from build123d import *

# Parameters (mm, degrees)
CROQUIS1_W     = 30
CROQUIS1_H     = 40
CROQUIS1_H_2   = 30
CROQUIS1_W_2   = 40
EXTRUIR1_DEPTH = 30
CROQUIS5_W     = 30
CROQUIS5_H     = 30
EXTRUIR4_DEPTH = 40
CROQUIS2_W     = 30
CROQUIS2_H     = 30
CROQUIS2_W_2   = 24
CROQUIS2_H_2   = 24
EXTRUIR2_DEPTH = 40
CROQUIS3_W     = 30
CROQUIS3_H     = 30
CROQUIS3_W_2   = 24
CROQUIS3_H_2   = 24
EXTRUIR3_DEPTH = 40
CROQUIS7_W     = 30
CROQUIS7_H     = 30
CROQUIS7_W_2   = 24
CROQUIS7_H_2   = 24
EXTRUIR5_DEPTH = 40
VACIADO1_T     = -2


with BuildPart() as part:
    # Croquis1 → Extruir1 (new body)
    with BuildSketch(Plane(origin=(0, 0, 0), x_dir=(1, 0, 0), z_dir=(0, 1, 0))):
        with Locations((0, 35)):
            Rectangle(CROQUIS1_W, CROQUIS1_H)
        Rectangle(CROQUIS1_W, CROQUIS1_H_2)
        with Locations((35, 0)):
            Rectangle(CROQUIS1_W_2, CROQUIS1_H_2)
    extrude(amount=EXTRUIR1_DEPTH)

    # Croquis5 → Extruir4 (add)
    with BuildSketch(Plane.XZ):
        Rectangle(CROQUIS5_W, CROQUIS5_H)
    extrude(amount=EXTRUIR4_DEPTH)

    # Croquis2 → Extruir2 (cut)
    with BuildSketch(Plane(origin=(55, 0, 0), x_dir=(0, 0, -1), z_dir=(1, 0, 0))):
        with Locations((0, 15)):
            Rectangle(CROQUIS2_W, CROQUIS2_H)
        with Locations((0, 15)):
            Rectangle(CROQUIS2_W_2, CROQUIS2_H_2, mode=Mode.SUBTRACT)
    extrude(amount=-EXTRUIR2_DEPTH, mode=Mode.SUBTRACT)

    # Croquis3 → Extruir3 (cut)
    with BuildSketch(Plane(origin=(0, 0, -55), x_dir=(-1, 0, 0), z_dir=(0, 0, -1))):
        with Locations((0, 15)):
            Rectangle(CROQUIS3_W, CROQUIS3_H)
        with Locations((0, 15)):
            Rectangle(CROQUIS3_W_2, CROQUIS3_H_2, mode=Mode.SUBTRACT)
    extrude(amount=-EXTRUIR3_DEPTH, mode=Mode.SUBTRACT)

    # Croquis7 → Extruir5 (cut)
    with BuildSketch(Plane.XZ.offset(40)):
        Rectangle(CROQUIS7_W, CROQUIS7_H)
        Rectangle(CROQUIS7_W_2, CROQUIS7_H_2, mode=Mode.SUBTRACT)
    extrude(amount=-EXTRUIR5_DEPTH, mode=Mode.SUBTRACT)

    # Vaciado1
    vaciado1_openings = [part.faces().sort_by_distance(p)[0] for p in [
        (55, 15, 0),
        (0, 15, -55),
        (0, -40, 0),
    ]]
    offset(amount=VACIADO1_T, openings=vaciado1_openings, kind=Kind.INTERSECTION)


solid = part.part
CAD build for the part. Positions are in the model's coordinates, mm. A direction names the side the tool comes from. Round coordinates to 2 decimals unless told otherwise and drop trailing zeros. Order: outer loops, then holes, each group sorted by start corner. A loop starts at its lowest first (then second) coordinate and runs counter-clockwise, first axis right, second up. Notation, with made-up numbers: M 27,83.25 L 55,83.25 A29 cw 55,113.25 Z; hole C 87.25,73.25 d10. An arc over 180 degrees is marked long. Use one line per item in the form item = value.
Q1. Saw through at D-D on z = 2. Give the cut face in (x, y).
Recorded:
outline = M -15,0 L -12,0 L -12,-40 L -10,-40 L -10,2 L -13,2 L -13,28 L 13,28 L 13,25 L 55,25 L 55,27 L 15,27 L 15,30 L -15,30 Z; M 10,-40 L 12,-40 L 12,0 L 15,0 L 15,3 L 55,3 L 55,5 L 13,5 L 13,2 L 10,2 Z
Q2. Saw through at C-C on x = 45. Give the cut face in (y, z).
Recorded:
outline = M 3,-12 L 27,-12 L 27,12 L 3,12 Z; hole M 5,-10 L 25,-10 L 25,10 L 5,10 Z
Q3. Flat gauge pins, fed straight in: P1, Ø10, axis at x = -2.5, y = -13.5, coming from the +Z side; P2, Ø12, axis at y = -14, z = -12, coming from the +X side; P3, Ø10, axis at x = 26.5, z = -2, coming from the +Y side. Where does each tip first touch, or does it go through?
Recorded:
P1 = 12
P2 = 12
P3 = 27
Q4. Saw through at B-B on z = -51. Give the cut face in (x, y), then the cut area to 3 significant figures.
Recorded:
outline = M -12,3 L 12,3 L 12,27 L -12,27 Z; hole M -10,5 L 10,5 L 10,25 L -10,25 Z
area = 176 mm^2
Q5. Saw through at A-A on x = 5.5. Give the cut face in (y, z), then the cut area to 3 significant figures.
Recorded:
outline = M -40,-12 L 0,-12 L 0,-15 L 3,-15 L 3,-55 L 5,-55 L 5,-13 L 2,-13 L 2,-10 L -40,-10 Z; M -40,10 L 2,10 L 2,13 L 28,13 L 28,-13 L 25,-13 L 25,-55 L 27,-55 L 27,-15 L 30,-15 L 30,15 L 0,15 L 0,12 L -40,12 Z
area = 464 mm^2
Q6. Probe L1, parallel to X at y = -34, z = 6; L2, parallel to Y at x = 2, z = -21. List the from-to ranges inside material, lowest first.
Recorded:
L1 = -12 to -10, 10 to 12
L2 = 3 to 5, 25 to 27
Q7. Which spindle directions (+Z, -Z, +X, -X, +Y, -Y) get a long thin tool onto all of the face, cutting with end or side? Do faces 4 (the flat face through (0, 3, -35)), 5 (the flat face through (-10, 15, -34)), 6 (the flat face through (12, -20, 0)). Say none if no direction does.
Recorded:
face_4 = -Z, +X, -X, -Y
face_5 = -Z
face_6 = +Z, -Z, +X, -Y
Q8. Two-plate mould, pull along X, no slides. Class faces 1 (the flat face through (-13, 15, 0)), 2 (the flat face through (55, 14.8, -10.5)), 3 (the flat face through (-15, 15, 0)): +X half, -X half, draft (parallel to the pull), parting line (faces both ways), or undercut.
Recorded:
face_1 = undercut
face_2 = +X half
face_3 = -X half
